Geometry: see drawing. Coordinates: mm, zero at the bounding-box minimum. Round coordinates to 2 decimals unless told otherwise and drop trailing zeros. Loops run counter-clockwise (first coordinate to the right, second up) from the corner with the lowest first, then second, coordinate; pieces in that order, holes last. Notation, with made-up numbers: M 68.5,-15 L 98.5,-15 A12 ccw 98.5,-3 Z; hole C 32.5,11 d2. An arc over 180 degrees is marked long. Answer as a JSON object with one key per item and string values.
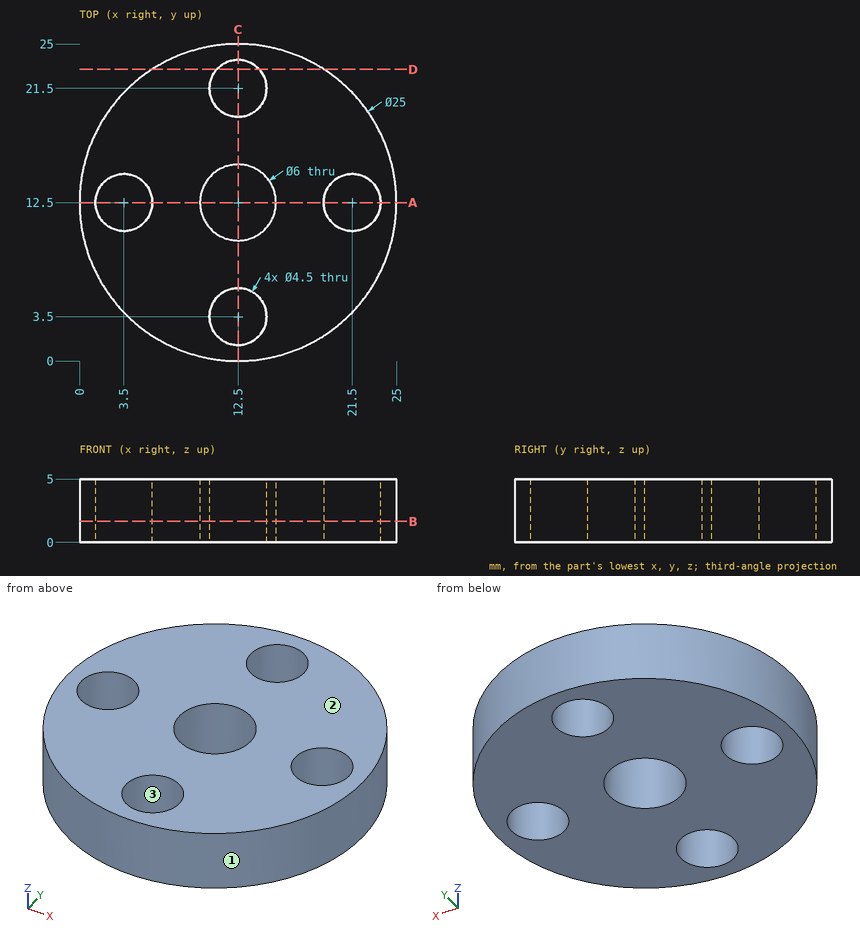
1) Ray query, line 1 (Y direction, x = 12.5, z = 2.05); line 2 (Y direction, x = 11.5, z = 4.55); line 3 (X direction, y = 3.5, z = 2.35). Return the intervals inside material, ascending.
Results:
{"line 1": "0 to 1.25, 5.75 to 9.5, 15.5 to 19.25, 23.75 to 25", "line 2": "0.04 to 1.48, 5.52 to 9.67, 15.33 to 19.48, 23.52 to 24.96", "line 3": "3.83 to 10.25, 14.75 to 21.17"}
2) Pull-direction query (X, two-part tool) for the marked faces 1, 2 and 3; classes: +X half, -X half, draft (parallel to the pull), parting line (faces both ways), or undercut.
Results:
{"face 1": "parting line", "face 2": "draft", "face 3": "undercut"}
3) Section query B-B (z = 1.65). Return the cut outline in (x, y), and give its area (3 significant figures).
Results:
{"outline": "C 12.5,12.5 d25; hole C 3.5,12.5 d4.5; hole C 12.5,12.5 d6; hole C 12.5,3.5 d4.5; hole C 12.5,21.5 d4.5; hole C 21.5,12.5 d4.5", "area": "399 mm2"}
4) Pin query (flat end, axial travel): P1, Ø5, axis at x = 21.5, y = 12.5, coming from the -Z side; P2, Ø2, axis at x = 10, z = 0.5, coming from the -Y side; P3, Ø4, axis at x = 3.5, y = 12.5, coming from the -Z side; P4, Ø2, axis at y = 21.5, z = 1, coming from the -X side. Return the tip coordinate at first contact, or that it passes through.
Results:
{"P1": "z = 0", "P2": "y = 0.09", "P3": "through", "P4": "x = 2.9"}
5) Section query D-D (y = 23). Return the cut outline in (x, z), and give its area (3 significant figures).
Results:
{"outline": "M 5.72,0 L 10.82,0 L 10.82,5 L 5.72,5 Z; M 14.18,0 L 19.28,0 L 19.28,5 L 14.18,5 Z", "area": "51.1 mm2"}
6) Section query A-A (y = 12.5). Return the cut outline in (x, z).
Results:
{"outline": "M 0,0 L 1.25,0 L 1.25,5 L 0,5 Z; M 5.75,0 L 9.5,0 L 9.5,5 L 5.75,5 Z; M 15.5,0 L 19.25,0 L 19.25,5 L 15.5,5 Z; M 23.75,0 L 25,0 L 25,5 L 23.75,5 Z"}
